```python
from build123d import *

# Parameters (mm, degrees)
F0_W     = 24
F0_H     = 158
F1_DEPTH = 24
F2_W     = 24
F2_H     = 24
F3_DEPTH = 202
F4_W     = 24
F4_H     = 24
F5_DEPTH = 720
F6_W     = 24
F6_H     = 24
F7_DEPTH = 280


with BuildPart() as f1:
    # F0 (on Front) → F1 (new body)
    with BuildSketch(Plane.XZ):
        Polygon((-330.027685374, 158.2459368452), (-354.027685374, 158.2459368452), (-354.027685374, 110.2459368452), (-354.027685374, 86.2459368452), (365.972314626, 86.2459368452), (365.972314626, 98.2459368452), (341.972314626, 98.2459368452), (-330.027685374, 98.2459368452), align=None)
        Polygon((365.972314626, 110.2459368452), (365.972314626, 158.2459368452), (341.972314626, 158.2459368452), (341.972314626, 98.2459368452), (365.972314626, 98.2459368452), align=None)
        Polygon((-330.027685374, 74.2459368452), (-354.027685374, 74.2459368452), (-354.027685374, 62.2459368452), (-354.027685374, -83.7540631548), (-330.027685374, -83.7540631548), align=None)
        with Locations((353.972314626, -4.7540631548)):
            Rectangle(F0_W, F0_H)
        Polygon((365.972314626, 86.2459368452), (-354.027685374, 86.2459368452), (-354.027685374, 74.2459368452), (-330.027685374, 74.2459368452), (341.972314626, 74.2459368452), (365.972314626, 74.2459368452), align=None)
        Polygon((365.972314626, 182.2459368452), (-354.027685374, 182.2459368452), (-354.027685374, 158.2459368452), (-330.027685374, 158.2459368452), (341.972314626, 158.2459368452), (365.972314626, 158.2459368452), align=None)
        Polygon((-330.027685374, -83.7540631548), (-354.027685374, -83.7540631548), (-354.027685374, -107.7540631548), (365.972314626, -107.7540631548), (365.972314626, -83.7540631548), (341.972314626, -83.7540631548), align=None)
    extrude(amount=-F1_DEPTH)

    # F2 (on face) → F3 (join)
    with BuildSketch(Plane(origin=(0, 24, 0), x_dir=(-1, 0, 0), z_dir=(0, 1, 0))):
        with Locations((-353.972314626, 86.2459368452)):
            Rectangle(F2_W, F2_H)
        with Locations((-353.972314626, -95.7540631548)):
            Rectangle(F2_W, F2_H)
        with Locations((342.027685374, 170.2459368452)):
            Rectangle(F2_W, F2_H)
        with Locations((342.027685374, -95.7540631548)):
            Rectangle(F2_W, F2_H)
        with Locations((342.027685374, 86.2459368452)):
            Rectangle(F2_W, F2_H)
        with Locations((-353.972314626, 170.2459368452)):
            Rectangle(F2_W, F2_H)
    extrude(amount=F3_DEPTH)

    # F4 (on face) → F5 (join)
    with BuildSketch(Plane.YZ.offset(365.972314626)):
        with Locations((238, 86.2459368452)):
            Rectangle(F4_W, F4_H)
        with Locations((238, 170.2459368452)):
            Rectangle(F4_W, F4_H)
        with Locations((238, -95.7540631548)):
            Rectangle(F4_W, F4_H)
    extrude(amount=-F5_DEPTH)

    # F6 (on face) → F7 (join)
    with BuildSketch(Plane.XY.offset(182.2459368452)):
        with Locations((-342.027685374, 238)):
            Rectangle(F6_W, F6_H)
        with Locations((353.972314626, 238)):
            Rectangle(F6_W, F6_H)
    extrude(amount=-F7_DEPTH)


solid = f1.part
```
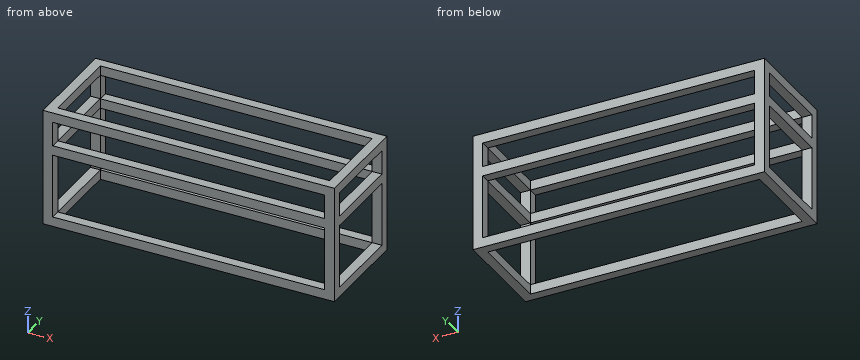
Geometry check sheet. Reference: the model listing, model coordinates, mm. Give positions to 0.01 mm unless a question says otherwise; leave off trailing zeros. Write each loop counter-clockwise with the first axis right and the second up, starting at its lowest first coordinate (ties: lowest second). Pieces come first, ordered by that corner, then holes. Notation, with made-up numbers: (30.5, 21.5) - (63.5, 21.5) arc R24 cw to (63.5, 33.5) - close; hole circle Ø2 at (32.25, 68). An arc over 180 degrees is marked (long way). Use a Markdown table: item, result.
Q1. Section check A-A, the plane y = 148. Enter the section's corners in (x, z), then the cut area to 3 significant figures.
Computed:
| item | result |
|---|---|
| outline | (-354.03, -107.75) - (-330.03, -107.75) - (-330.03, -83.75) - (-354.03, -83.75) - close; (-354.03, 74.25) - (-330.03, 74.25) - (-330.03, 98.25) - (-354.03, 98.25) - close; (-354.03, 158.25) - (-330.03, 158.25) - (-330.03, 182.25) - (-354.03, 182.25) - close; (341.97, -107.75) - (365.97, -107.75) - (365.97, -83.75) - (341.97, -83.75) - close; (341.97, 74.25) - (365.97, 74.25) - (365.97, 98.25) - (341.97, 98.25) - close; (341.97, 158.25) - (365.97, 158.25) - (365.97, 182.25) - (341.97, 182.25) - close |
| area | 3,460 mm² |
Q2. Section check C-C, the plane x = -37.5. Enter the section's corners in (y, z).
Computed:
| item | result |
|---|---|
| outline | (0, -107.75) - (24, -107.75) - (24, -83.75) - (0, -83.75) - close; (0, 74.25) - (24, 74.25) - (24, 98.25) - (0, 98.25) - close; (0, 158.25) - (24, 158.25) - (24, 182.25) - (0, 182.25) - close; (226, -107.75) - (250, -107.75) - (250, -83.75) - (226, -83.75) - close; (226, 74.25) - (250, 74.25) - (250, 98.25) - (226, 98.25) - close; (226, 158.25) - (250, 158.25) - (250, 182.25) - (226, 182.25) - close |
Q3. Thickness scan on L1, parallel to Y at x = -213.5, z = 77.5; L2, parallel to X at y = 12.5, z = 67.5. Record the ranges inside material, lowest first. Write a range as [from, to].
Computed:
| item | result |
|---|---|
| L1 | y = [0, 24], [226, 250] |
| L2 | x = [-354.03, -330.03], [341.97, 365.97] |
Q4. Section check B-B, the plane z = -14.5. Enter the section's corners in (x, y), then the cut area to 3 significant figures.
Computed:
| item | result |
|---|---|
| outline | (-354.03, 0) - (-330.03, 0) - (-330.03, 24) - (-354.03, 24) - close; (-354.03, 226) - (-330.03, 226) - (-330.03, 250) - (-354.03, 250) - close; (341.97, 0) - (365.97, 0) - (365.97, 24) - (341.97, 24) - close; (341.97, 226) - (365.97, 226) - (365.97, 250) - (341.97, 250) - close |
| area | 2,300 mm² |
